Verification items for the finished model (mm, model axes). A direction names the side the tool comes from. Coordinates: 2 decimals unless noted, no trailing zeros. Write each loop counter-clockwise with the first axis right and the second up, starting at its lowest first coordinate (ties: lowest second). Pieces come first, ordered by that corner, then holes.
```python
from build123d import *

# Parameters (mm, degrees)
F1_DEPTH = 14.5
F3_DEPTH = 1.5
F4_R     = 4.5
F5_DEPTH = 3
F6_R     = 3.5
F7_DEPTH = 3


with BuildPart() as f1:
    # F0 (on Right) → F1 (new body, symmetric)
    with BuildSketch(Plane.YZ):
        with BuildLine():
            Line((-5, 0), (-298, 0))
            Line((-298, 0), (-298, -3))
            Line((-298, -3), (-5, -3))
            ThreePointArc((-5, -3), (-3.585786, -3.585786), (-3, -5))
            Line((-3, -5), (-3, -208))
            Line((-3, -208), (0, -208))
            Line((0, -208), (0, -5))
            ThreePointArc((0, -5), (-1.464466, -1.464466), (-5, 0))
        make_face()
    extrude(amount=F1_DEPTH, both=True)

    # F2 (on Right) → F3 (join, symmetric)
    with BuildSketch(Plane.YZ):
        Polygon((-3, -150.343812), (-3, -127), (-209, -3), (-247.780849, -3), align=None)
    extrude(amount=F3_DEPTH, both=True)

    # F4 (on face) → F5 (cut)
    with BuildSketch(Plane(origin=(0, 0, 0), x_dir=(-1, 0, 0), z_dir=(0, 1, 0))):
        with Locations((0, -28.5)):
            Circle(F4_R)
        with Locations((0, -78.5)):
            Circle(F4_R)
        with Locations((0, -182.5)):
            Circle(F4_R)
    extrude(amount=-F5_DEPTH, mode=Mode.SUBTRACT)

    # F6 (on face) → F7 (cut)
    with BuildSketch(Plane.XY):
        with Locations((-5, -38.5)):
            Circle(F6_R)
        with Locations((4, -128.5)):
            Circle(F6_R)
        with Locations((0, -270)):
            Circle(F6_R)
    extrude(amount=-F7_DEPTH, mode=Mode.SUBTRACT)


solid = f1.part
```
1. Draft check along Y on faces 1 (the flat face through (0, -149, 0)), 2 (the flat face through (0, 0, -108)), 3 (the cylindrical face through (-5, -35, -1)). Enter one of: pulls with the +Y half, pulls with the -Y half, needs draft (parallel to the pull), parting line crosses it, or undercut.
2. Sectioned sample at A-A, the plane y = -270. Record the boundary of the cut face in (x, z), and give its area (3 significant figures).
3. Gauge pin test, flat ends, axial feed: P1, Ø11.5, axis at x = 0, z = -28.5, coming from the -Y side; P2, Ø10.5, axis at x = 0, z = -78.5, coming from the -Y side; P3, Ø14.5, axis at x = 1.5, z = -112, coming from the -Y side; P4, Ø5.5, axis at x = 0, z = -182.5, coming from the +Y side. Record the tip position at first contact, or that the pin passes through.
4. Sectioned sample at D-D, the plane y = -38.5. Record the boundary of the cut face in (x, z).
5. Sectioned sample at B-B, the plane z = -28.5. Record the boundary of the cut face in (x, y), and give its area (3 significant figures).
6. Material ranges on L1, parallel to Z at x = 0, y = -1.5; L2, parallel to Z at x = 0, y = -1.45; L3, parallel to X at y = -270, z = -1.75, recorded low to high.
7. Tool access check on faces 4 (the cylindrical face through (3.241, -131.917, -1.479)), 5 (the flat face through (-1.5, -117, -71)), 6 (the flat face through (1.5, -117, -71)). Record the directions out of +Z, -Z, +X, -X, +Y, -Y that give a thin tool (end or side, any length) a straight path to the whole face; none if there is none.
8. Sectioned sample at C-C, the plane z = -62.5. Record the boundary of the cut face in (x, y), and give its area (3 significant figures).
Outcome:
1. face 1: needs draft
1. face 2: pulls with the +Y half
1. face 3: undercut
2. outline: (-14.5, -3) - (-3.5, -3) - (-3.5, 0) - (-14.5, 0) - close; (3.5, -3) - (14.5, -3) - (14.5, 0) - (3.5, 0) - close
2. area: 66.0 mm2
3. P1: stops at y = -214.97
3. P2: stops at y = -131.08
3. P3: stops at y = -78.74
3. P4: passes through
4. outline: (-14.5, -3) - (-8.5, -3) - (-8.5, 0) - (-14.5, 0) - close; (-1.5, -128.97) - (1.5, -128.97) - (1.5, -105.63) - (-1.5, -105.63) - close; (-1.5, -3) - (14.5, -3) - (14.5, 0) - (-1.5, 0) - close
5. outline: (-14.5, -3) - (-4.5, -3) - (-4.5, 0) - (-14.5, 0) - close; (-1.5, -205.42) - (1.5, -205.42) - (1.5, -166.64) - (-1.5, -166.64) - close; (4.5, -3) - (14.5, -3) - (14.5, 0) - (4.5, 0) - close
5. area: 176 mm2
6. L1: z = -208 to -187, -178 to -83, -74 to -33, -24 to -1.43
6. L2: z = -208 to -187, -178 to -83, -74 to -33, -24 to -1.48
6. L3: x = -14.5 to -3.5, 3.5 to 14.5
7. face 4: +Z
7. face 5: -Z, -X, -Y
7. face 6: -Z, +X, -Y
8. outline: (-14.5, -3) - (14.5, -3) - (14.5, 0) - (-14.5, 0) - close; (-1.5, -148.93) - (1.5, -148.93) - (1.5, -110.15) - (-1.5, -110.15) - close
8. area: 203 mm2
